from build123d import *

# Parameters (mm, degrees)
SKETCH_1_W          = 15
SKETCH_1_H          = 5
SKETCH_1_R          = 0.85
EXTRUDE_1_DEPTH     = 2
SKETCH_2_W          = 6
SKETCH_2_H          = 6
EXTRUDE_3_DEPTH     = 6
CUT_EXTRUDE_2_DEPTH = 6
SKETCH_7_W          = 3.2
SKETCH_7_H          = 3.2
CUT_EXTRUDE_3_DEPTH = 2
SKETCH_10_W         = 6
SKETCH_10_H         = 6.172231081
SKETCH_10_W_2       = 3.2
SKETCH_10_H_2       = 3.2
EXTRUDE_4_DEPTH     = 5


with BuildPart() as part:
    # 草图1 → 凸台-拉伸1 (new body)
    with BuildSketch(Plane(origin=(0, 0, 0), x_dir=(1, 0, 0), z_dir=(0, 1, 0))):
        with Locations((7.5, 2.5)):
            Rectangle(SKETCH_1_W, SKETCH_1_H)
        with Locations(Location((3.25, 2.5, 0), (0, 0, 270))):
            Circle(SKETCH_1_R, mode=Mode.SUBTRACT)
        with Locations(Location((11.75, 2.5, 0), (0, 0, 90))):
            Circle(SKETCH_1_R, mode=Mode.SUBTRACT)
    extrude(amount=EXTRUDE_1_DEPTH)

    # 草图2 → 凸台-拉伸3 (add)
    with BuildSketch(Plane.XZ):
        with Locations((7.5, -2.5)):
            Rectangle(SKETCH_2_W, SKETCH_2_H)
    extrude(amount=EXTRUDE_3_DEPTH)

    # 草图6 → 切除-拉伸2 (cut)
    with BuildSketch(Plane(origin=(0, 0, -5.5), x_dir=(-1, 0, 0), z_dir=(0, 0, -1))):
        Polygon((-10.5, -0.2), (-10.5, -6), (-8.388972641, -6), align=None)
    extrude(amount=-CUT_EXTRUDE_2_DEPTH, mode=Mode.SUBTRACT)

    # 草图7 → 切除-拉伸3 (cut)
    with BuildSketch(Plane(origin=(9.336012087, -3.398030507, 0), x_dir=(0, 0, -1), z_dir=(0.9396926207859104, -0.3420201433256631, 0))):
        with Locations((2.5, 0.317157441)):
            Rectangle(SKETCH_7_W, SKETCH_7_H)
    extrude(amount=-CUT_EXTRUDE_3_DEPTH, mode=Mode.SUBTRACT)

    # 草图10 → 凸台-拉伸4 (add)
    with BuildSketch(Plane(origin=(9.336012087, -3.398030507, 0), x_dir=(0, 0, -1), z_dir=(0.9396926207859104, -0.3420201433256631, 0))):
        with Locations((2.5, 0.31715744)):
            Rectangle(SKETCH_10_W, SKETCH_10_H)
        with Locations((2.5, 0.317157441)):
            Rectangle(SKETCH_10_W_2, SKETCH_10_H_2, mode=Mode.SUBTRACT)
    extrude(amount=EXTRUDE_4_DEPTH)


solid = part.part
Work out the finished part from the listing and answer in its coordinate system (mm). A direction names the side the tool comes from. Give positions to 0.01 mm unless a question says otherwise; leave off trailing zeros. Write each loop counter-clockwise with the first axis right and the second up, starting at its lowest first coordinate (ties: lowest second). Pieces come first, ordered by that corner, then holes.
Q1. A tool of negligible diameter and unlimited length cuts with its end or side. For faces 5 (the face through (6, -6, -2)), 6 (the face through (15, 1, -2)), 7 (the face through (13, 0, -3)), from which of +Z, -Z, +X, -X, +Y, -Y can it reach the whole face along a straight path? Write none if from no direction.
Answer:
face 5: +Z, -Z, -X, -Y
face 6: +Z, -Z, +X, +Y
face 7: +Z, -Z, +X
Q2. The part is cut by section D-D on y = 1.25. Give the vertices of the cut face in (x, z), and give its area (3 significant figures).
Answer:
outline: (0, -5) - (15, -5) - (15, 0) - (0, 0) - close; hole circle Ø1.7 at (3.25, -2.5); hole circle Ø1.7 at (11.75, -2.5)
area: 70.5 mm2
Q3. For a pull along X with two mould halves and no side action, classify faces 1 (the face through (11, -4, -0.9)), 2 (the face through (7, 2, -3)), 3 (the face through (12.816, -1.043, -2.458)), 4 (the face through (10.705, -6.843, -2.458)) as released by +X, released by -X, zero draft, split by the parting line, or undercut.
Answer:
face 1: undercut
face 2: zero draft
face 3: released by +X
face 4: released by -X
Q4. The part is cut by section B-B on z = -2.5. Give the vertices of the cut face in (x, y), and give its area (3 significant figures).
Answer:
outline: (0, 0) - (2.4, 0) - (2.4, 2) - (0, 2) - close; (4.1, 0) - (4.5, 0) - (4.5, -6) - (8.39, -6) - (13.09, -7.71) - (13.6, -6.31) - (7.02, -3.92) - (8.11, -0.91) - (14.69, -3.31) - (15.2, -1.91) - (10.5, -0.2) - (10.5, 0) - (10.9, 0) - (10.9, 2) - (4.1, 2) - close; (12.6, 0) - (15, 0) - (15, 2) - (12.6, 2) - close
area: 61.5 mm2
Q5. Straight lines are drawn through the part: L1, parallel to X at y = 0.75, z = -2.5; L2, parallel to Z at x = 11.75, y = 0.8; L3, parallel to Y at x = 11.25, z = -3.95. For each, find the intervals that lie inside material, in ascending order.
Answer:
L1: x = 0 to 2.4, 4.1 to 10.9, 12.6 to 15
L2: z = -5 to -3.35, -1.65 to 0
L3: y = -7.04 to -5.46, -2.05 to -0.47, 0 to 2
Q6. Given pin 1 (1 mm diameter, centred on x = 12, z = -2, fed in from -Y); pin 2 (1.3 mm diameter, centred on x = 1.5, z = -2.5, fed in from -Y); pin 3 (0.6 mm diameter, centred on x = 7, y = 1, fed in from +Z), each flat-ended and moving along its own axis, determine where each tip first touches the part or whether it passes through.
Answer:
pin 1: stops at y = -7.5
pin 2: stops at y = 0
pin 3: stops at z = 0
Q7. The part is cut by section C-C on x = 11.5. Give the vertices of the cut face in (y, z), and give its area (3 significant figures).
Answer:
outline: (-7.13, -5.5) - (-0.56, -5.5) - (-0.56, 0.5) - (-7.13, 0.5) - close; (0, -5) - (2, -5) - (2, -3.31) - (0, -3.31) - close; (0, -1.69) - (2, -1.69) - (2, 0) - (0, 0) - close; hole (-5.55, -4.1) - (-2.15, -4.1) - (-2.15, -0.9) - (-5.55, -0.9) - close
area: 35.3 mm2
Q8. The part is cut by section A-A on x = 3.25. Give the vertices of the cut face in (y, z), and give its area (3 significant figures).
Answer:
outline: (0, -5) - (2, -5) - (2, -3.35) - (0, -3.35) - close; (0, -1.65) - (2, -1.65) - (2, 0) - (0, 0) - close
area: 6.60 mm2
